Autodesk Inventor part; units mm, degrees
ref_plane "p1_XY" through (0, 0, 3.175) normal (1, 0, 0) x (0, 0, -1)
ref_plane "p1_YZ" through (0, 0, 3.175) normal (0, 0, -1) x (0, 1, 0)
ref_plane "p1_ZX" through (0, 0, 3.175) normal (0, 1, 0) x (1, 0, 0)
sketch "Sketch_1" plane through (0, 0, 0) normal (0, 0, 1) x (1, 0, 0)
  line L0 (8.763, 0) -> (-8.763, 0)
  line L1 (-8.763, 0) -> (-8.763, 2.794)
  line L2 (-8.763, 2.794) -> (-8.382, 3.175)
  line L3 (-8.382, 3.175) -> (-7.5565, 3.175)
  line L4 (-7.5565, 3.175) -> (-7.5565, 2.667)
  line L5 (-7.5565, 2.667) -> (-6.35, 2.667)
  line L6 (-6.35, 2.667) -> (-6.35, 3.175)
  line L7 (-6.35, 3.175) -> (6.35, 3.175)
  line L8 (6.35, 3.175) -> (6.35, 2.667)
  line L9 (6.35, 2.667) -> (7.5565, 2.667)
  line L10 (7.5565, 2.667) -> (7.5565, 3.175)
  line L11 (7.5565, 3.175) -> (8.382, 3.175)
  line L12 (8.382, 3.175) -> (8.763, 2.794)
  line L13 (8.763, 2.794) -> (8.763, 0)
  line L14 (8.763, 0) -> (-8.763, 0)
revolve "Revolution1" add sketch "Sketch_1" angle 360 about axis through (8.763, 0, 0) along (1, 0, 0)
ref_plane "p1_XY" through (0, 0, 3.175) normal (1, 0, 0) x (0, 0, -1)
ref_plane "p1_YZ" through (0, 0, 3.175) normal (0, 0, -1) x (0, 1, 0)
ref_plane "p1_ZX" through (0, 0, 3.175) normal (0, 1, 0) x (1, 0, 0)
ref_plane "p2_XY" through (0, 0, -3.175) normal (1, 0, 0) x (0, 0, -1)
ref_plane "p2_YZ" through (0, 0, -3.175) normal (0, 0, -1) x (0, 1, 0)
ref_plane "p2_ZX" through (0, 0, -3.175) normal (0, 1, 0) x (1, 0, 0)
ref_plane "pin_XY" through (0, 0, 0) normal (1, 0, 0) x (0, 0, -1)
ref_plane "pin_YZ" through (0, 0, 0) normal (0, 0, -1) x (0, 1, 0)
ref_plane "pin_ZX" through (0, 0, 0) normal (0, 1, 0) x (1, 0, 0)
ref_plane "rr1_XY" through (6.9532, 0, 0) normal (1, 0, 0) x (0, 0, -1)
ref_plane "rr1_YZ" through (6.9532, 0, 0) normal (0, 0, -1) x (0, 1, 0)
ref_plane "rr1_ZX" through (6.9532, 0, 0) normal (0, 1, 0) x (1, 0, 0)
ref_plane "rr2_XY" through (-6.9532, 0, 0) normal (1, 0, 0) x (0, 0, -1)
ref_plane "rr2_YZ" through (-6.9532, 0, 0) normal (0, 0, -1) x (0, 1, 0)
ref_plane "rr2_ZX" through (-6.9532, 0, 0) normal (0, 1, 0) x (1, 0, 0)
ref_plane "w21_XY" through (8.763, 0, 0) normal (0, 1, 0) x (1, 0, 0)
ref_plane "w21_YZ" through (8.763, 0, 0) normal (1, 0, 0) x (0, 0, -1)
ref_plane "w21_ZX" through (8.763, 0, 0) normal (0, 0, -1) x (0, 1, 0)
ref_plane "w22_XY" through (-8.763, 0, 0) normal (0, 1, 0) x (1, 0, 0)
ref_plane "w22_YZ" through (-8.763, 0, 0) normal (1, 0, 0) x (0, 0, -1)
ref_plane "w22_ZX" through (-8.763, 0, 0) normal (0, 0, -1) x (0, 1, 0)
properties part number "D-8381" material "Aluminum 6061"
The model under review builds one solid part; all positions refer to its coordinate system, in mm. A direction names the side the tool comes from. Round coordinates to 2 decimals unless told otherwise and drop trailing zeros. Order: outer loops, then holes, each group sorted by start corner. A loop starts at its lowest first (then second) coordinate and runs counter-clockwise, first axis right, second up. Notation, with made-up numbers: (76, -29.5) -> (81, -29.5) arc R33 cw to (81, 5.5) -> close; hole circle Ø2 at (28, 87.5). An arc over 180 degrees is marked (long way). Write item = value, one per line. Start each with the question number.
Item 1: Consider section B-B on x = 1. Write out the cut boundary in (y, z) (3 decimals).
Item 2: Clearance check with a flat-ended pin moving along its axis: pin 1 Ø3 at (x, y) = (2.5, 1.5) entering from -Z (3 decimals). State where the tip first meets the part, or that it passes through.
Item 3: For line 1 along Z through (x, y) = (-7.5, 0); line 2 along X through (y, z) = (-1.75, -2.5); line 3 along X through (y, z) = (-1.5, 2.5), list the stretches that pass through material, from the lowest coordinate up.
Item 4: For faces 4 (the face through (-6.35, -2, 2)), 5 (the face through (7.98, -0.69, -3.1)), list the 3-axis set-ups (+Z, -Z, +X, -X, +Y, -Y) from which the entire face can be reached by the end or side of a thin tool; tool diameter is ignored.
Item 5: Consider section C-C on x = -6.75. Write out the cut boundary in (y, z), plus the area to 3 significant figures.
Item 6: Mouldability with a two-part tool opening along X and no side actions: class faces 1 (the face through (-8.763, 0, 0)), 2 (the face through (-7.96, -0.69, -3.1)), 3 (the face through (6.35, -2, 2)) as released by +X, released by -X, zero draft, split by the parting line, or undercut.
Conclusion:
q1.outline = circle Ø6.35 at (0, 0)
q2.pin_1 = -3.175
q3.line_1 = -2.67 to 2.67
q3.line_2 = -8.51 to -7.56, -6.35 to 6.35, 7.56 to 8.51
q3.line_3 = -8.64 to -7.56, -6.35 to 6.35, 7.56 to 8.64
q4.face_4 = none
q4.face_5 = +X, -X
q5.outline = circle Ø5.33 at (0, 0)
q5.area = 22.3 mm2
q6.face_1 = released by -X
q6.face_2 = zero draft
q6.face_3 = undercut
